Design review of the part built by this model. Coordinates are the model's own, in mm. A direction names the side the tool comes from. Give positions to 0.01 mm unless a question says otherwise; leave off trailing zeros. Order: outer loops, then holes, each group sorted by start corner. A loop starts at its lowest first (then second) coordinate and runs counter-clockwise, first axis right, second up. Notation, with made-up numbers: (43.25, -9) -> (90.25, -9) arc R23 ccw to (90.25, 22) -> close; hole circle Ø2 at (65, -16). An arc over 180 degrees is marked (long way). Return JSON: item names as keys, results as strings.
```python
from build123d import *

# Parameters (mm, degrees)
ESQUISSE2_W             = 6
ESQUISSE2_H             = 6
BOSS_EXTRU_1_DEPTH      = 6
ESQUISSE4_W             = 4
ESQUISSE4_H             = 4
ENL_V_MAT_EXTRU_1_DEPTH = 3.1
CHANFREIN1_SIZE         = 0.03


with BuildPart() as part:
    # Esquisse2 → Boss.-Extru.1 (new body)
    with BuildSketch(Plane(origin=(0, 0, 0), x_dir=(1, 0, 0), z_dir=(0, 1, 0))):
        Rectangle(ESQUISSE2_W, ESQUISSE2_H)
    extrude(amount=BOSS_EXTRU_1_DEPTH)

    # Esquisse4 → Enlèv. mat.-Extru.1 (cut)
    with BuildSketch(Plane(origin=(0, 6, 0), x_dir=(1, 0, 0), z_dir=(0, 1, 0))):
        Rectangle(ESQUISSE4_W, ESQUISSE4_H)
    extrude(amount=-ENL_V_MAT_EXTRU_1_DEPTH, mode=Mode.SUBTRACT)

    # Chanfrein1
    chanfrein1_edges = [part.edges().sort_by_distance(p)[0] for p in [
        (-3, 6, 0),
        (2, 2.9, 0),
        (2, 4.45, -2),
        (0, 6, 3),
        (0, 2.9, 2),
        (2, 4.45, 2),
        (-2, 2.9, 0),
        (-2, 4.45, 2),
        (0, 2.9, -2),
        (-2, 4.45, -2),
        (2, 6, 0),
        (0, 6, -2),
        (-2, 6, 0),
        (0, 6, 2),
        (3, 6, 0),
        (3, 3, 3),
        (-3, 3, 3),
        (-3, 3, -3),
        (3, 3, -3),
        (0, 6, -3),
    ]]
    chamfer(chanfrein1_edges, length=CHANFREIN1_SIZE)


solid = part.part
```
Item 1: For pin 1 (2 mm diameter, centred on x = 0.5, z = -1, fed in from -Y); pin 2 (1.2 mm diameter, centred on x = 0, z = 1, fed in from +Y), all flat-tipped, find the tip position at first contact; note any pin that passes through.
Result set:
{"pin 1": "stops at y = 0", "pin 2": "stops at y = 2.9"}
Item 2: Wall thickness on L1, parallel to Z at x = 1, y = 5.4; L2, parallel to Y at x = 1.75, z = 1: over which ranges is each line inside the solid? List them lowest first. Write a range as [from, to].
Result set:
{"L1": "z = [-3, -2], [2, 3]", "L2": "y = [0, 2.9]"}
Item 3: Mouldability with a two-part tool opening along X and no side actions: class faces 1 (the face through (0, 2.9, 0)), 2 (the face through (-3, 3, 0)), 3 (the face through (-2.7, 6, 0)) as released by +X, released by -X, zero draft, split by the parting line, or undercut.
Result set:
{"face 1": "undercut", "face 2": "released by -X", "face 3": "zero draft"}
Item 4: Machinability: for faces 4 (the face through (0, 0, 0)), 5 (the face through (0, 4, -2)), which of the approach directions +Z, -Z, +X, -X, +Y, -Y give a long, thin tool a straight path to every point of the face, cutting with its end or side? Answer none if there is none.
Result set:
{"face 4": "+Z, -Z, +X, -X, -Y", "face 5": "+Y"}
Item 5: Add section A-A (y = 5.2). Give the boundary of the cut face in (x, z).
Result set:
{"outline": "(-3, -2.97) -> (-2.97, -3) -> (2.97, -3) -> (3, -2.97) -> (3, 2.97) -> (2.97, 3) -> (-2.97, 3) -> (-3, 2.97) -> close; hole (-2, -1.97) -> (-1.97, -2) -> (1.97, -2) -> (2, -1.97) -> (2, 1.97) -> (1.97, 2) -> (-1.97, 2) -> (-2, 1.97) -> close"}
Item 6: Add section C-C (x = -1.5). Give the boundary of the cut face in (y, z).
Result set:
{"outline": "(0, -3) -> (5.97, -3) -> (6, -2.97) -> (6, -2.03) -> (5.97, -2) -> (2.93, -2) -> (2.9, -1.97) -> (2.9, 1.97) -> (2.93, 2) -> (5.97, 2) -> (6, 2.03) -> (6, 2.97) -> (5.97, 3) -> (0, 3) -> close"}
Item 7: Add section B-B (z = -1). Give the boundary of the cut face in (x, y), plus the area to 3 significant figures.
Result set:
{"outline": "(-3, 0) -> (3, 0) -> (3, 5.97) -> (2.97, 6) -> (2.03, 6) -> (2, 5.97) -> (2, 2.93) -> (1.97, 2.9) -> (-1.97, 2.9) -> (-2, 2.93) -> (-2, 5.97) -> (-2.03, 6) -> (-2.97, 6) -> (-3, 5.97) -> close", "area": "23.6 mm^2"}
